Build history of the part. All positions in model axes, mm. Round coordinates to 2 decimals unless told otherwise and drop trailing zeros. Order: outer loops, then holes, each group sorted by start corner. A loop starts at its lowest first (then second) coordinate and runs counter-clockwise, first axis right, second up. Notation, with made-up numbers: (69.5, 34.25) -> (76.5, 34.25) arc R28 cw to (76.5, 57.25) -> close; hole circle Ø5 at (48, 44). An arc over 180 degrees is marked (long way). Answer as a JSON object with one key per item and string values.
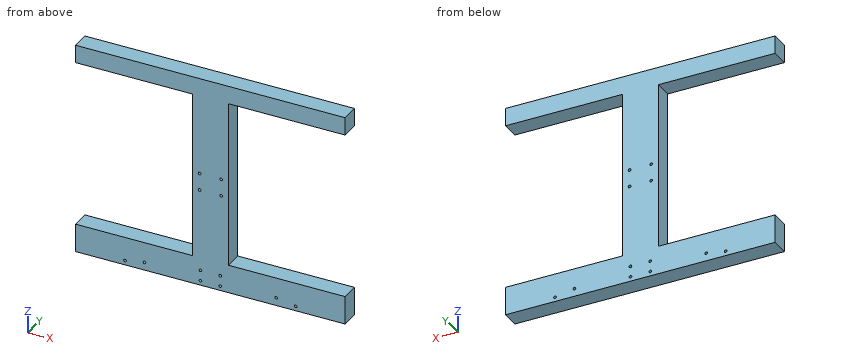
Autodesk Inventor part; units mm, degrees
ref_plane "YZ Plane" through (0, 0, 0) normal (1, 0, 0) x (0, 1, 0)
ref_plane "XZ Plane" through (0, 0, 0) normal (0, 1, 0) x (-1, 0, 0)
ref_plane "XY Plane" through (0, 0, 0) normal (0, 0, 1) x (1, 0, 0)
sketch "草图1" plane through (0, 0, 0) normal (0, 1, 0) x (-1, 0, 0)
  line L0 (16.7619, 206.381) -> (-23.2381, 206.381)
  line L1 (-23.2381, 206.381) -> (-23.2381, -31.619)
  line L2 (-23.2381, -31.619) -> (16.7619, -31.619)
  line L3 (16.7619, -31.619) -> (16.7619, 206.381)
  point P0 (0, 0)
  dimension "d0" = 40
  dimension "d1" = 238
extrude "拉伸1" add sketch "草图1" along normal blind 20
sketch "草图2" plane through (23.2381, 0, 206.381) normal (1, 0, 0) x (0, 0, -1)
  line L0 (238, 20) -> (0, 20)
  line L1 (238, 0) -> (0, 0)
  line L2 (0, 20) -> (20, 20)
  line L3 (20, 20) -> (20, 0)
  line L4 (20, 0) -> (0, 0)
  line L5 (0, 0) -> (0, 20)
  point P0 (206.381, 0)
  dimension "d4" = 20
extrude "拉伸2" add sketch "草图2" along normal blind 20
sketch "草图5" plane through (-16.7619, 0, -31.619) normal (-1, 0, 0) x (0, 0, 1)
  line L0 (0, 0) -> (238, 0)
  line L1 (218, 20) -> (0, 20)
  line L2 (238, 0) -> (218, 0)
  line L3 (218, 0) -> (218, 20)
  line L4 (218, 20) -> (238, 20)
  line L5 (238, 20) -> (238, 0)
  point P0 (31.619, 0)
extrude "拉伸3" add sketch "草图5" along normal blind 20
sketch "草图6" plane through (-16.7619, 0, -31.619) normal (-1, 0, 0) x (0, 0, 1)
  line L0 (0, 0) -> (0, 20)
  line L1 (218, 0) -> (0, 0)
  line L2 (0, 20) -> (20, 20)
  line L3 (20, 20) -> (20, 0)
  line L4 (20, 0) -> (0, 0)
  line L5 (0, 0) -> (0, 20)
  point P0 (31.619, 0)
  dimension "d9" = 20
extrude "拉伸4" add sketch "草图6" along normal blind 20
sketch "草图7" plane through (23.2381, 0, -31.619) normal (1, 0, 0) x (0, 0, -1)
  line L0 (0, 0) -> (0, 20)
  line L1 (-20, 0) -> (-218, 0)
  line L2 (0, 20) -> (-20, 20)
  line L3 (-20, 20) -> (-20, 0)
  line L4 (-20, 0) -> (0, 0)
  line L5 (0, 0) -> (0, 20)
  point P0 (-31.619, 0)
extrude "拉伸5" add sketch "草图7" along normal blind 20
sketch "草图8" plane through (0, 20, 0) normal (0, 1, 0) x (1, 0, 0)
  line L0 (23.2381, -186.381) -> (23.2381, 11.619)
  line L1 (-16.7619, 11.619) -> (-16.7619, -186.381)
  circle A0 centre (-8.7619, -96.881) radius 1.5
  circle A1 centre (-8.7619, -77.881) radius 1.5
  circle A2 centre (15.2381, -96.881) radius 1.5
  circle A3 centre (15.2381, -77.881) radius 1.5
  point P0 (0, 0)
extrude "拉伸6" cut sketch "草图8" against normal through all
sketch "草图9" plane through (0, 20, 0) normal (0, 1, 0) x (1, 0, 0)
  line L0 (-36.7619, 31.619) -> (43.2381, 31.619)
  line L1 (3.2381, 31.619) -> (3.2381, -247.5925)
  line L2 (3.2381, 31.619) -> (153.2381, 31.619)
  line L3 (3.2381, 31.619) -> (-146.7619, 31.619)
  line L4 (-146.7619, 31.619) -> (-146.7619, 11.619)
  line L5 (-16.7619, 11.619) -> (-36.7619, 11.619)
  line L6 (-146.7619, 11.619) -> (153.2381, 11.619)
  line L7 (153.2381, 11.619) -> (153.2381, 31.619)
  line L8 (-146.7619, -186.381) -> (153.2381, -186.381)
  line L9 (153.2381, -186.381) -> (153.2381, -206.381)
  line L10 (43.2381, -206.381) -> (-36.7619, -206.381)
  line L11 (153.2381, -206.381) -> (-146.7619, -206.381)
  line L12 (-146.7619, -206.381) -> (-146.7619, -186.381)
  point P0 (0, 0)
  dimension "d20" = 150
  dimension "d21" = 150
extrude "拉伸7" add sketch "草图9" against normal blind 20
sketch "草图10" plane through (0, 20, 0) normal (0, 1, 0) x (1, 0, 0)
  line L0 (3.2381, 42.6) -> (3.2381, -82.4296)
  line L1 (-146.7619, 31.619) -> (153.2381, 31.619)
  line L2 (3.2381, 31.619) -> (3.2381, 26.619)
  line L3 (3.2381, 26.619) -> (14.2381, 26.619)
  line L4 (14.2381, 26.619) -> (-7.7619, 26.619)
  circle A0 centre (-7.7619, 26.619) radius 1.5
  circle A1 centre (14.2381, 26.619) radius 1.5
  line L5 (14.2381, 26.619) -> (14.2381, 14.619)
  circle A2 centre (14.2381, 14.619) radius 1.5
  line L6 (-7.7619, 26.619) -> (-7.7619, 14.619)
  circle A3 centre (-7.7619, 14.619) radius 1.5
  point P0 (0, 0)
  dimension "d27" = 5
  dimension "d28" = 11
  dimension "d29" = 22
  dimension "d30" = 3
  dimension "d31" = 3
  dimension "d32" = 12
  dimension "d33" = 3
  dimension "d34" = 12
  dimension "d35" = 3
extrude "拉伸8" cut sketch "草图10" against normal through all
sketch "草图12" plane through (0, 20, 0) normal (0, 1, 0) x (1, 0, 0)
  line L0 (-146.7619, 31.619) -> (-91.7619, 31.619)
  line L1 (-91.7619, 31.619) -> (-91.7619, 26.619)
  circle A0 centre (-91.7619, 26.619) radius 1.5
  line L2 (3.2381, 31.619) -> (3.2381, -27.4763)
  line L3 (98.2381, 31.619) -> (98.2381, 26.619)
  circle A1 centre (98.2381, 26.619) radius 1.5
  line L4 (-91.7619, 26.619) -> (-70.0961, 22.7988)
  circle A2 centre (14.2381, 26.619) radius 1.5
  circle A3 centre (-7.7619, 26.619) radius 1.5
  circle A4 centre (-70.0961, 22.7988) radius 1.5
  circle A5 centre (76.5723, 22.7988) radius 1.5
  point P0 (0, 0)
  dimension "d43" = 55
  dimension "d50" = 22
  dimension "d51" = 3
  dimension "d58" = 100
  dimension "d59" = 5
extrude "拉伸9" cut sketch "草图12" against normal through all contours A0 L4 L1 | A4 | L1 L4 A0 | A1 | A5
sketch "草图13" plane through (23.2381, 0, 186.381) normal (1, 0, 0) x (0, 0, -1)
  line L0 (0, 20) -> (198, 20)
  line L1 (198, 20) -> (186.381, 20)
  line L2 (186.381, 20) -> (186.381, 0)
  line L3 (186.381, 0) -> (198, 0)
  line L4 (198, 0) -> (198, 20)
extrude "拉伸10" add sketch "草图13" along normal blind 130 and the other way blind 5
sketch "草图14" plane through (-16.7619, 0, 186.381) normal (-1, 0, 0) x (0, 0, 1)
  line L0 (-198, 20) -> (-198, 0)
  line L1 (-186.381, 0) -> (-186.381, 20)
  line L2 (-198, 0) -> (-186.381, 0)
  line L3 (-186.381, 0) -> (-186.381, 20)
  line L4 (-186.381, 20) -> (-198, 20)
  line L5 (-198, 20) -> (-198, 0)
  point P0 (-197.5, 20)
extrude "拉伸11" add sketch "草图14" along normal blind 130
equation "\"折弯半径\" = 厚度"
equation "\"折弯释压宽度\" = 厚度"
equation "\"折弯释压深度\" = 0.5 * 厚度"
equation "\"拐角释压尺寸\" = 4 * 厚度"
equation "\"最小余量\" = 2 * 厚度"
equation "\"过渡半径\" = 折弯半径"
equation "\"Jacobi半径尺寸\" = 折弯半径"
equation "\"间隙大小\" = 厚度"
properties part number "固定架"
1) Cut at A-A, the plane x = -78.5. Give the cut face in (y, z).
Checked values:
{"outline": "(0, -31.62) -> (20, -31.62) -> (20, 0) -> (0, 0) -> close; (0, 186.38) -> (20, 186.38) -> (20, 206.38) -> (0, 206.38) -> close"}
2) Cut at C-C, the plane z = 84. Give the cut face in (x, y).
Checked values:
{"outline": "(-16.76, 0) -> (23.24, 0) -> (23.24, 20) -> (-16.76, 20) -> close"}
3) Probe L1, parallel to Z at x = 120.5, y = 11.5; L2, parallel to X at y = 5.75, z = -14; L3, parallel to X at y = 7.25, z = 180.5. List the from-to ranges inside material, lowest first. Write a range as from..to.
Checked values:
{"L1": "z = -31.62..0, 186.38..206.38", "L2": "x = -146.76..-9.13, -6.4..12.87, 15.6..153.24", "L3": "x = -16.76..23.24"}
4) Flat gauge pins, fed straight in: pin 1 Ø1 at (y, z) = (3.5, 62.5) entering from -X; pin 2 Ø10 at (y, z) = (9, 105.5) entering from +X. Where does each tip first touch, or does it go through?
Checked values:
{"pin 1": "stops at x = -16.76", "pin 2": "stops at x = 23.24"}
5) Cut at B-B, the plane y = 17. Count the separate pieces of the cut face and the enclosed holes in it, plus the area to 3 significant figures.
Checked values:
{"separate pieces": "1", "enclosed holes": "12", "area": "22,900 mm²"}
